Here's how the part is built. I have some questions about the finished solid (model axes, mm). Face numbers are marked on the shaded views. A direction names the side the tool comes from. Give positions to 0.01 mm unless a question says otherwise; leave off trailing zeros. Loops run counter-clockwise (first coordinate to the right, second up) from the corner with the lowest first, then second, coordinate; pieces in that order, holes last. Notation, with made-up numbers: (-14, -9.75) - (31, -9.75) arc R20 ccw to (31, 9.25) - close; hole circle Ø3 at (-38, -7.75). An arc over 180 degrees is marked (long way). Use a Markdown table: item, result.
from build123d import *

# Parameters (mm, degrees)
BOSS_EXTRUDE1_START = 30
SKETCH1_W           = 16.4
SKETCH1_H           = 14.4
SKETCH1_W_2         = 12.4
SKETCH1_H_2         = 10.4
BOSS_EXTRUDE1_DEPTH = 15
BOSS_EXTRUDE2_START = 30
BOSS_EXTRUDE2_DEPTH = 15


with BuildPart() as part:
    # Sketch1 → Boss-Extrude1 (new body)
    with BuildSketch(Plane(origin=(0, 0, 0), x_dir=(0, 0, -1), z_dir=(1, 0, 0)).offset(BOSS_EXTRUDE1_START)):
        Rectangle(SKETCH1_W, SKETCH1_H)
        Rectangle(SKETCH1_W_2, SKETCH1_H_2, mode=Mode.SUBTRACT)
    extrude(amount=BOSS_EXTRUDE1_DEPTH)

    # Sketch2 → Boss-Extrude2 (add)
    with BuildSketch(Plane(origin=(0, 0, 0), x_dir=(0, 0, -1), z_dir=(1, 0, 0)).offset(BOSS_EXTRUDE2_START)):
        with BuildLine():
            Line((-3.924283374, 7.2), (3.924283374, 7.2))
            ThreePointArc((3.924283374, 7.2), (8.2, 0), (3.924283374, -7.2))
            Line((3.924283374, -7.2), (-3.924283374, -7.2))
            ThreePointArc((-3.924283374, -7.2), (-8.2, 0), (-3.924283374, 7.2))
        make_face()
        with BuildLine():
            Line((-3.376388603, 5.2), (3.376388603, 5.2))
            ThreePointArc((3.376388603, 5.2), (6.2, 0), (3.376388603, -5.2))
            Line((3.376388603, -5.2), (-3.376388603, -5.2))
            ThreePointArc((-3.376388603, -5.2), (-6.2, 0), (-3.376388603, 5.2))
        make_face(mode=Mode.SUBTRACT)
    extrude(amount=-BOSS_EXTRUDE2_DEPTH)


solid = part.part
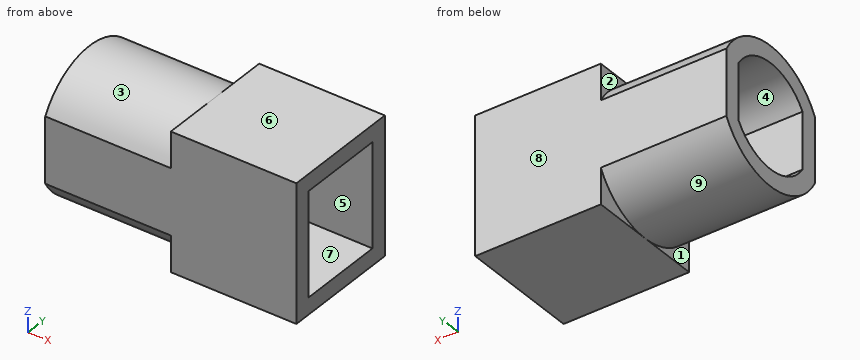
(1) Suppose I cut it at D-D on x = 28.25. Write out the boundary of the cut face in (y, z).
A:
| item | result |
|---|---|
| outline | (-7.2, -3.92) arc R8.2 ccw to (7.2, -3.92) - (7.2, 3.92) arc R8.2 ccw to (-7.2, 3.92) - close; hole (-5.2, -3.38) arc R6.2 ccw to (5.2, -3.38) - (5.2, 3.38) arc R6.2 ccw to (-5.2, 3.38) - close |
(2) If I drill on line 1 (Z direction, x = 41.25, y = -0.25); line 2 (Y direction, x = 30, z = 1.5); line 3 (Y direction, x = 27, z = 4.25), over which ranges is the centre line in solid material (lowest first)?
A:
| item | result |
|---|---|
| line 1 | -8.2 to -6.2, 6.2 to 8.2 |
| line 2 | -7.2 to -5.2, 5.2 to 7.2 |
| line 3 | -7.01 to -4.51, 4.51 to 7.01 |
(3) Suppose I cut it at B-B on z = 0.5. Write out the boundary of the cut face in (x, y).
A:
| item | result |
|---|---|
| outline | (15, -7.2) - (45, -7.2) - (45, -5.2) - (15, -5.2) - close; (15, 5.2) - (45, 5.2) - (45, 7.2) - (15, 7.2) - close |
(4) We'd pull the mould along Y, two halves only. Please class the marked faces 6, 7, 8 and 9: pulls with the +Y half, pulls with the -Y half, needs draft (parallel to the pull), parting line crosses it, or undercut.
A:
| item | result |
|---|---|
| face 6 | needs draft |
| face 7 | undercut |
| face 8 | pulls with the +Y half |
| face 9 | parting line crosses it |
(5) On a 3-axis mill with a long thin cutter (end or side, diameter ignored), from which of +Z, -Z, +X, -X, +Y, -Y can I reach the whole of each face in a straight line? I mean the marked faces 1, 2, 3, 4 and 5. Say none if no direction works.
A:
| item | result |
|---|---|
| face 1 | -Z, -X, -Y |
| face 2 | +Z, -X, +Y |
| face 3 | +Z, -X |
| face 4 | +X, -X |
| face 5 | +X |
(6) Suppose I cut it at A-A on x = 34. Write out the boundary of the cut face in (y, z).
A:
| item | result |
|---|---|
| outline | (-7.2, -8.2) - (7.2, -8.2) - (7.2, 8.2) - (-7.2, 8.2) - close; hole (-5.2, -6.2) - (5.2, -6.2) - (5.2, 6.2) - (-5.2, 6.2) - close |
(7) Will these pins go through, and if not, where does the flat tip stop? pin 1 (5 mm diameter, centred on x = 25, y = 4.5, fed in from +Z); pin 2 (0.8 mm diameter, centred on y = 3.5, z = 5, fed in from +X).
A:
| item | result |
|---|---|
| pin 1 | z = 7.95 |
| pin 2 | x = 30 |
